from build123d import *

# Parameters (mm, degrees)
SKETCH_1_W      = 52
SKETCH_1_H      = 41
EXTRUDE_1_DEPTH = 2
F_3_0MM_1_D     = 3.2
F_3_0MM_1_DEPTH = 2
F_3_0MM_1_TIP   = 0.96137699


with BuildPart() as part:
    # 草图1 → 凸台-拉伸1 (new body)
    with BuildSketch(Plane.XY):
        Polygon((35.75, 47.5), (35.75, 50.5), (-35.75, 50.5), (-35.75, 47.5), (-35.75, -47.5), (35.75, -47.5), align=None)
        with Locations((0, -22)):
            Rectangle(SKETCH_1_W, SKETCH_1_H, mode=Mode.SUBTRACT)
    extrude(amount=EXTRUDE_1_DEPTH)

    # Ø3.0mm 暗销孔1
    with Locations(Plane(origin=(68.159346192, -140.5, 0), x_dir=(-1, 0, 0), z_dir=(0, 0, -1))):
        with Locations((80.907068169, 161.379417443), (55.907068169, 161.379417443)):
            Hole(F_3_0MM_1_D / 2, depth=F_3_0MM_1_DEPTH)
            with Locations((0, 0, -(F_3_0MM_1_DEPTH + F_3_0MM_1_TIP / 2))):  # 118° drill point
                Cone(0, F_3_0MM_1_D / 2, F_3_0MM_1_TIP, mode=Mode.SUBTRACT)


solid = part.part
Input: part model. Units: mm. Frame: model coordinates. A direction names the side the tool comes from. Round coordinates to 2 decimals unless told otherwise and drop trailing zeros. Write each loop counter-clockwise with the first axis right and the second up, starting at its lowest first coordinate (ties: lowest second). Pieces come first, ordered by that corner, then holes.
1) Cut plane C-C (z = 1.1). Return the cut outline in (x, y).
2) Ray query, L1, parallel to Y at x = 12.5, z = 1.35; L2, parallel to Y at x = 7, z = 1.75; L3, parallel to X at y = -25, z = 0.65. Return the intervals inside material, ascending.
3) Draft query along Y for faces 1 (the flat face through (-1, -47.5, 1)), 2 (the flat face through (1, 50.5, 1)), 3 (the flat face through (-1, 13, 2)), 4 (the cylindrical face through (-11.27, 20.27, 1.01)). Return one class per face: pulls with the +Y half, pulls with the -Y half, needs draft (parallel to the pull), parting line crosses it, or undercut.
4) Cut plane A-A (y = -24). Return the cut outline in (x, z).
5) Reachability of faces 5 (the flat face through (-35.75, 2, 1)), 6 (the flat face through (0, -1.5, 1)) from +Z, -Z, +X, -X, +Y, -Y: full face, straight path, thin tool, end or side. Return the list, or none.
6) Cut plane B-B (x = -19.5). Return the cut outline in (y, z), then the cut area to 3 significant figures.
Geometry says:
1. outline: (-35.75, -47.5) - (35.75, -47.5) - (35.75, 50.5) - (-35.75, 50.5) - close; hole (-26, -42.5) - (26, -42.5) - (26, -1.5) - (-26, -1.5) - close; hole circle Ø3.2 at (-12.75, 20.88); hole circle Ø3.2 at (12.25, 20.88)
2. L1: y = -47.5 to -42.5, -1.5 to 19.3, 22.46 to 50.5
2. L2: y = -47.5 to -42.5, -1.5 to 50.5
2. L3: x = -35.75 to -26, 26 to 35.75
3. face 1: pulls with the -Y half
3. face 2: pulls with the +Y half
3. face 3: needs draft
3. face 4: undercut
4. outline: (-35.75, 0) - (-26, 0) - (-26, 2) - (-35.75, 2) - close; (26, 0) - (35.75, 0) - (35.75, 2) - (26, 2) - close
5. face 5: +Z, -Z, -X, +Y, -Y
5. face 6: +Z, -Z
6. outline: (-47.5, 0) - (-42.5, 0) - (-42.5, 2) - (-47.5, 2) - close; (-1.5, 0) - (50.5, 0) - (50.5, 2) - (-1.5, 2) - close
6. area: 114 mm2
